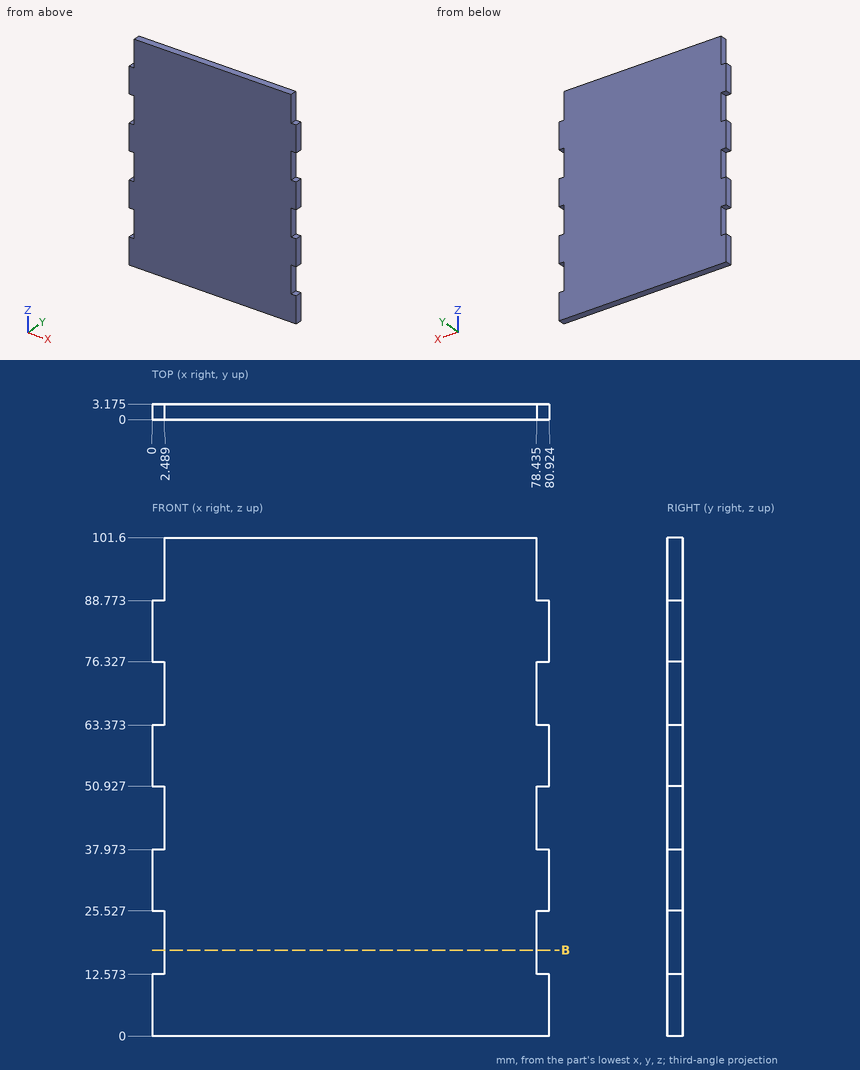
Job drawing, mm, ordinate dimensions from the low corner. One solid piece. Give positions to 0.01 mm unless a question says otherwise; leave off trailing zeros. Order: outer loops, then holes, each group sorted by start corner. A loop starts at its lowest first (then second) coordinate and runs counter-clockwise, first axis right, second up. Notation, with made-up numbers: M -9,30.25 L 19,30.25 A22 cw 19,63.25 Z; hole C -9,66 d9. An arc over 180 degrees is marked long. Put each result on its own line as item: value. Start each with the question number.
(1) Pin check, flat tips, straight feed: pin 1 Ø1 at (y, z) = (1, 67.5) entering from -X; pin 2 Ø1.2 at (x, y) = (1.5, 1) entering from +Z. Stop position of each tip, or through.
(2) Drill centre line: L1, parallel to X at y = 1.6, z = 67 (1 decimal). Where is it in solid material? Low to high. Write a range as [from, to].
(3) Band-saw the part on B-B on z = 17.5. Give the cut face in (x, y) (1 decimal), then the cut area to 3 significant figures.
Results below:
1. pin 1: stops at x = 2.49
1. pin 2: stops at z = 88.77
2. L1: x = [2.5, 78.4]
3. outline: M 2.5,0 L 78.4,0 L 78.4,3.2 L 2.5,3.2 Z
3. area: 241 mm2
